```python
from build123d import *

# Parameters (mm, degrees)
SKETCH_1_R          = 9
SKETCH_1_R_2        = 7
EXTRUDE_1_DEPTH     = 1
EXTRUDE_START       = -1
SKETCH_2_R          = 0.8
EXTRUDE_2_DEPTH     = 1
SKETCH_3_W          = 6.510588585
SKETCH_3_H          = 2.3
CUT_EXTRUDE_1_DEPTH = 15.201320361
FILLET_1_R          = 0.5


with BuildPart() as part:
    # 草图1 → 凸台-拉伸1 (new body)
    with BuildSketch(Plane(origin=(0, 0, 0), x_dir=(1, 0, 0), z_dir=(0, 1, 0))):
        with Locations(Location((0, 0, 0), (0, 0, 270))):
            Circle(SKETCH_1_R)
        with Locations(Location((0, 0, 0), (0, 0, 270))):
            Circle(SKETCH_1_R_2, mode=Mode.SUBTRACT)
    extrude(amount=EXTRUDE_1_DEPTH)

    # 草图2 → 凸台-拉伸2 (add)
    # profile 1 of 2: a face of its own
    with BuildSketch(Plane(origin=(0, 1, 0), x_dir=(1, 0, 0), z_dir=(0, 1, 0)).offset(EXTRUDE_START)):
        with BuildLine():
            Line((10.939721203, 1.15), (8.926225406, 1.15))
            ThreePointArc((8.926225406, 1.15), (8.427566507, 3.158500083), (7.483314774, 5))
            Line((7.483314774, 5), (9.797958971, 5))
            ThreePointArc((9.797958971, 5), (10.546016772, 3.127543804), (10.939721203, 1.15))
        make_face()
        with Locations(Location((9.7, 2.769537095, 0), (0, 0, 270))):
            Circle(SKETCH_2_R, mode=Mode.SUBTRACT)
    # profile 2 of 2: a face of its own
    with BuildSketch(Plane(origin=(0, 1, 0), x_dir=(1, 0, 0), z_dir=(0, 1, 0)).offset(EXTRUDE_START)):
        with BuildLine():
            Line((10.939721203, -1.15), (8.926225406, -1.15))
            ThreePointArc((8.926225406, -1.15), (8.427566507, -3.158500083), (7.483314774, -5))
            Line((7.483314774, -5), (9.797958971, -5))
            ThreePointArc((9.797958971, -5), (10.546016772, -3.127543804), (10.939721203, -1.15))
        make_face()
        with Locations(Location((9.7, -2.769537095, 0), (0, 0, 270))):
            Circle(SKETCH_2_R, mode=Mode.SUBTRACT)
    extrude(amount=EXTRUDE_2_DEPTH)

    # 草图3 → 切除-拉伸1 (cut, through all)
    with BuildSketch(Plane(origin=(0, 1, 0), x_dir=(1, 0, 0), z_dir=(0, 1, 0))):
        with Locations((7.684426911, 0)):
            Rectangle(SKETCH_3_W, SKETCH_3_H)
    extrude(amount=-CUT_EXTRUDE_1_DEPTH, mode=Mode.SUBTRACT)

    # 圆角1
    fillet_1_edges = [part.edges().sort_by_distance(p)[0] for p in [
        (10.939721203, 0.5, -1.15),
        (9.797958971, 0.5, -5),
        (9.797958971, 0.5, 5),
        (10.939721203, 0.5, 1.15),
    ]]
    fillet(fillet_1_edges, radius=FILLET_1_R)


solid = part.part
```
The listing builds one solid part. Answer for the finished solid, in the listing's coordinates (mm). A direction names the side the tool comes from. Round coordinates to 2 decimals unless told otherwise and drop trailing zeros. Write each loop counter-clockwise with the first axis right and the second up, starting at its lowest first coordinate (ties: lowest second). Pieces come first, ordered by that corner, then holes. Notation, with made-up numbers: (71, -4) -> (116, -4) arc R32 cw to (116, 28) -> close; hole circle Ø3 at (66, -21.75). An arc over 180 degrees is marked (long way). Use CSV: the item, a comma, the result in double quotes. Start each with the question number.
(1) Section A-A on x = 0 is taken. Give the vertices of the cut face in (y, z), then the cut area to 3 significant figures.
(2) This flat-tipped pin is pushed along its axis until it touches: pin 1 (0.5 mm diameter, centred on x = 9, y = 0.5, fed in from -Z). Where does it stop, or does it pass through?
(3) Which of the six approach directions +Z, -Z, +X, -X, +Y, -Y give full straight-line access (tool end or side, diameter ignored) to faces 1 (the face through (8.5, 0.5, 5)), 2 (the face through (8.6, 0.5, 1.15)), 3 (the face through (8.5, 0.5, -5))?
(4) Section D-D on z = 0 is taken. Give the vertices of the cut face in (x, y), then the cut area to 3 significant figures.
(5) Section B-B on y = 0.55 is taken. Give the vertices of the cut face in (x, z), then the cut area to 3 significant figures.
(6) Section C-C on z = 5.75 is taken. Give the vertices of the cut face in (x, y), then the cut area to 3 significant figures.
(7) The mould has two halves that part along X. Classify faces 4 (the face through (8.92, 0.49, 2.6)), 5 (the face through (-8.994, 0.493, -0.322)), 6 (the face through (7, 0, -2)): released by +X, released by -X, zero draft, split by the parting line, or undercut.
(8) Consider L1, parallel to Z at x = 9.5, y = 0.8; L2, parallel to X at y = 0.7, z = 2.5; L3, parallel to X at y = 0.7, z = 4. Determine where each line is inside the solid, lowest interval first. Write a range as from..to.
A:
1,outline,"(0, -9) -> (1, -9) -> (1, -7) -> (0, -7) -> close; (0, 7) -> (1, 7) -> (1, 9) -> (0, 9) -> close"
1,area,"4.00 mm²"
2,pin 1,"stops at z = -5"
3,face 1,"+Z, +X, +Y, -Y"
3,face 2,"+X, +Y, -Y"
3,face 3,"-Z, +X, +Y, -Y"
4,outline,"(-9, 0) -> (-7, 0) -> (-7, 1) -> (-9, 1) -> close"
4,area,"2.00 mm²"
5,outline,"(6.9, -1.15) arc R7 cw (long way) to (6.9, 1.15) -> (10.37, 1.15) arc R0.5 ccw to (10.86, 1.73) arc R11 ccw to (9.94, 4.71) arc R0.5 ccw to (9.49, 5) -> (7.48, 5) arc R9 ccw (long way) to (7.48, -5) -> (9.49, -5) arc R0.5 ccw to (9.94, -4.71) arc R11 ccw to (10.86, -1.73) arc R0.5 ccw to (10.37, -1.15) -> close; hole circle Ø1.6 at (9.7, -2.77); hole circle Ø1.6 at (9.7, 2.77)"
5,area,"108 mm²"
6,outline,"(-6.92, 0) -> (-3.99, 0) -> (-3.99, 1) -> (-6.92, 1) -> close; (3.99, 0) -> (6.92, 0) -> (6.92, 1) -> (3.99, 1) -> close"
6,area,"5.86 mm²"
7,face 4,"undercut"
7,face 5,"split by the parting line"
7,face 6,"zero draft"
8,L1,"z = -5..-3.54, -1.99..-1.15, 1.15..1.99, 3.54..5"
8,L2,"x = -8.65..-6.54, 6.54..8.95, 10.45..10.71"
8,L3,"x = -8.06..-5.74, 5.74..10.25"
